Read the model definition and answer for the solid it produces. Units are mm, in the model's axes. A direction names the side the tool comes from. Give positions to 0.01 mm unless a question says otherwise; leave off trailing zeros. Loops run counter-clockwise (first coordinate to the right, second up) from the corner with the lowest first, then second, coordinate; pieces in that order, holes last.
(1) Find section B-B, the plane y = 31.5. Write down the section's boundary in (x, z).
(2) Each of these flat-tipped pins is pushed along its axis until it touches: P1, Ø1.5, axis at y = -5, z = 1, coming from the +X side; P2, Ø1.2, axis at x = 0, y = 14, coming from the -Z side; P3, Ø1, axis at x = -21, z = 1.5, coming from the +Y side; P4, Ø1.7, axis at x = 14, y = 0, coming from the +Z side. Where does it stop, or does it pass through?
(3) Find section A-A, the plane z = 0.8. State how many separate pieces and enclosed holes the cut face has, then the cut area to 3 significant figures.
(4) Find section C-C, the plane x = -41. Write down the section's boundary in (y, z), then the cut area to 3 significant figures.
(5) Straight lines are drawn through the part: probe 1 along Y at (x, z) = (0, 1.3); probe 2 along X at (y, z) = (-9, 2.3); probe 3 along Y at (x, z) = (-14, 0.9). For each, find the intervals that lie inside material, in ascending order.
(6) Which of the six approach directions +Z, -Z, +X, -X, +Y, -Y give full straight-line access (tool end or side, diameter ignored) to faces 1 (the face through (10, 1, 3)), 2 (the face through (24, -10.5, 2))?
(7) Determine the mould class of faces 3 (the face through (-10.3, -46.37, 1.48)), 4 (the face through (10, 1, 0)), 5 (the face through (-25.5, -7, 2)) for opening direction X: pulls with the +X half, pulls with the -X half, needs draft (parallel to the pull), parting line crosses it, or undercut.
```python
from build123d import *

# Parameters (mm, degrees)
CROQUIS1_R              = 47.5
CROQUIS1_R_2            = 2.5
CROQUIS1_R_3            = 0.75
SALIENTE_EXTRUIR1_DEPTH = 3
CROQUIS2_W              = 3
CROQUIS2_H              = 8
CORTAR_EXTRUIR1_DEPTH   = 4


with BuildPart() as part:
    # Croquis1 → Saliente-Extruir1 (new body)
    with BuildSketch(Plane.XY):
        Circle(CROQUIS1_R)
        Circle(CROQUIS1_R_2, mode=Mode.SUBTRACT)
        with Locations((0, -14)):
            Circle(CROQUIS1_R_3, mode=Mode.SUBTRACT)
        with Locations((-14, 0)):
            Circle(CROQUIS1_R_3, mode=Mode.SUBTRACT)
        with Locations((0, 14)):
            Circle(CROQUIS1_R_3, mode=Mode.SUBTRACT)
        with Locations((14, 0)):
            Circle(CROQUIS1_R_3, mode=Mode.SUBTRACT)
    extrude(amount=SALIENTE_EXTRUIR1_DEPTH)

    # Croquis2 → Cortar-Extruir1 (cut, through all)
    with BuildSketch(Plane.XY.offset(3)):
        with Locations((24, 6.5)):
            Rectangle(CROQUIS2_W, CROQUIS2_H)
        with Locations((24, -6.5)):
            Rectangle(CROQUIS2_W, CROQUIS2_H)
        with Locations((-24, -6.5)):
            Rectangle(CROQUIS2_W, CROQUIS2_H)
        with Locations((-24, 6.5)):
            Rectangle(CROQUIS2_W, CROQUIS2_H)
    extrude(amount=-CORTAR_EXTRUIR1_DEPTH, mode=Mode.SUBTRACT)


solid = part.part
```
Entries:
1. outline: (-35.55, 0) - (35.55, 0) - (35.55, 3) - (-35.55, 3) - close
2. P1: stops at x = 47.31
2. P2: passes through
2. P3: stops at y = 42.85
2. P4: stops at z = 3
3. separate pieces: 1
3. enclosed holes: 9
3. area: 6,970 mm2
4. outline: (-23.98, 0) - (23.98, 0) - (23.98, 3) - (-23.98, 3) - close
4. area: 144 mm2
5. probe 1: y = -47.5 to -14.75, -13.25 to -2.5, 2.5 to 13.25, 14.75 to 47.5
5. probe 2: x = -46.64 to -25.5, -22.5 to 22.5, 25.5 to 46.64
5. probe 3: y = -45.39 to -0.75, 0.75 to 45.39
6. face 1: +Z, +X, -X, +Y, -Y
6. face 2: +Z, -Z
7. face 3: parting line crosses it
7. face 4: needs draft
7. face 5: undercut
